Build history of the part. All positions in model axes, mm. Coordinates: 2 decimals unless noted, no trailing zeros. Loops run counter-clockwise (first coordinate to the right, second up) from the corner with the lowest first, then second, coordinate; pieces in that order, holes last.
Item 1: Cut at A-A (x = 9). List the corners of the cut face in (y, z), and give its area (3 significant figures).
Item 2: Cut at B-B (y = 22). List the corners of the cut face in (x, z), and give its area (3 significant figures).
Item 3: Drill centre lines: line 1 along Y through (x, z) = (82.5, 1.05); line 2 along Y through (x, z) = (9, 0.7); line 3 along X through (y, z) = (12, 1.3). Where is each one in solid material? Low to high.
Item 4: Flat gauge pin, fed straight in: pin 1 (6.5 mm diameter, centred on x = 82.5, y = 109, fed in from -Z). Where does the tip first touch, or does it go through?
Item 5: Mould opens along X. For faces 1 (the face through (0.86, 6.9, 1.48)), 2 (the face through (84, 14, 1)), 3 (the face through (8.46, 96.56, 1.48)), 4 (the face through (164.1, 6.86, 1.48)) say: released by +X, released by -X, zero draft, split by the parting line, or undercut.
from build123d import *

# Parameters (mm, degrees)
SKETCH_1_W          = 165
SKETCH_1_H          = 118.00212
SKETCH_1_R          = 2.5
EXTRUDE_1_DEPTH     = 3
FILLET_1_R          = 3
CUT_EXTRUDE_START   = -10
CUT_EXTRUDE_1_DEPTH = 10
FILLET_2_R          = 3


with BuildPart() as part:
    # ｽｹｯﾁ1 → ﾎﾞｽ - 押し出し1 (new body)
    with BuildSketch(Plane.XY):
        with Locations((82.5, 59.00106)):
            Rectangle(SKETCH_1_W, SKETCH_1_H)
        with Locations((82.5, 109.00212)):
            Circle(SKETCH_1_R, mode=Mode.SUBTRACT)
        with Locations((9, 99.00212)):
            Circle(SKETCH_1_R, mode=Mode.SUBTRACT)
        with Locations(Location((9, 22, 0), (0, 0, 180))):
            Circle(SKETCH_1_R, mode=Mode.SUBTRACT)
        with Locations(Location((82.5, 12, 0), (0, 0, 180))):
            Circle(SKETCH_1_R, mode=Mode.SUBTRACT)
        with Locations(Location((156, 99.00212, 0), (0, 0, 180))):
            Circle(SKETCH_1_R, mode=Mode.SUBTRACT)
        with Locations((156, 22)):
            Circle(SKETCH_1_R, mode=Mode.SUBTRACT)
    extrude(amount=EXTRUDE_1_DEPTH)

    # ﾌｨﾚｯﾄ1
    fillet_1_edges = [part.edges().sort_by_distance(p)[0] for p in [
        (0, 0, 1.5),
        (0, 118.00212, 1.5),
        (165, 118.00212, 1.5),
        (165, 0, 1.5),
    ]]
    fillet(fillet_1_edges, radius=FILLET_1_R)

    # ｽｹｯﾁ3 → ｶｯﾄ - 押し出し1 (cut)
    with BuildSketch(Plane(origin=(0, 0, 0), x_dir=(-1, 0, 0), z_dir=(0, 0, -1)).offset(CUT_EXTRUDE_START)):
        with BuildLine():
            Line((-162, 0), (-82.5, 0))
            Line((-82.5, 0), (-82.5, 6))
            Line((-82.5, 6), (-165, 6))
            Line((-165, 6), (-165, 3))
            ThreePointArc((-165, 3), (-164.121320344, 0.878679656), (-162, 0))
        make_face()
        with BuildLine():
            Line((-82.5, 6), (-82.5, 0))
            Line((-82.5, 0), (-3, 0))
            ThreePointArc((-3, 0), (-0.878679656, 0.878679656), (0, 3))
            Line((0, 3), (0, 6))
            Line((0, 6), (-82.5, 6))
        make_face()
    extrude(amount=CUT_EXTRUDE_1_DEPTH, mode=Mode.SUBTRACT)

    # ﾌｨﾚｯﾄ2
    fillet_2_edges = [part.edges().sort_by_distance(p)[0] for p in [
        (165, 6, 1.5),
        (0, 6, 1.5),
    ]]
    fillet(fillet_2_edges, radius=FILLET_2_R)


solid = part.part
Filled sheet:
1. outline: (6, 0) - (19.5, 0) - (19.5, 3) - (6, 3) - close; (24.5, 0) - (96.5, 0) - (96.5, 3) - (24.5, 3) - close; (101.5, 0) - (118, 0) - (118, 3) - (101.5, 3) - close
1. area: 306 mm2
2. outline: (0, 0) - (6.5, 0) - (6.5, 3) - (0, 3) - close; (11.5, 0) - (153.5, 0) - (153.5, 3) - (11.5, 3) - close; (158.5, 0) - (165, 0) - (165, 3) - (158.5, 3) - close
2. area: 465 mm2
3. line 1: y = 6 to 9.5, 14.5 to 106.5, 111.5 to 118
3. line 2: y = 6 to 19.5, 24.5 to 96.5, 101.5 to 118
3. line 3: x = 0 to 80, 85 to 165
4. pin 1: stops at z = 0
5. face 1: released by -X
5. face 2: undercut
5. face 3: undercut
5. face 4: released by +X
